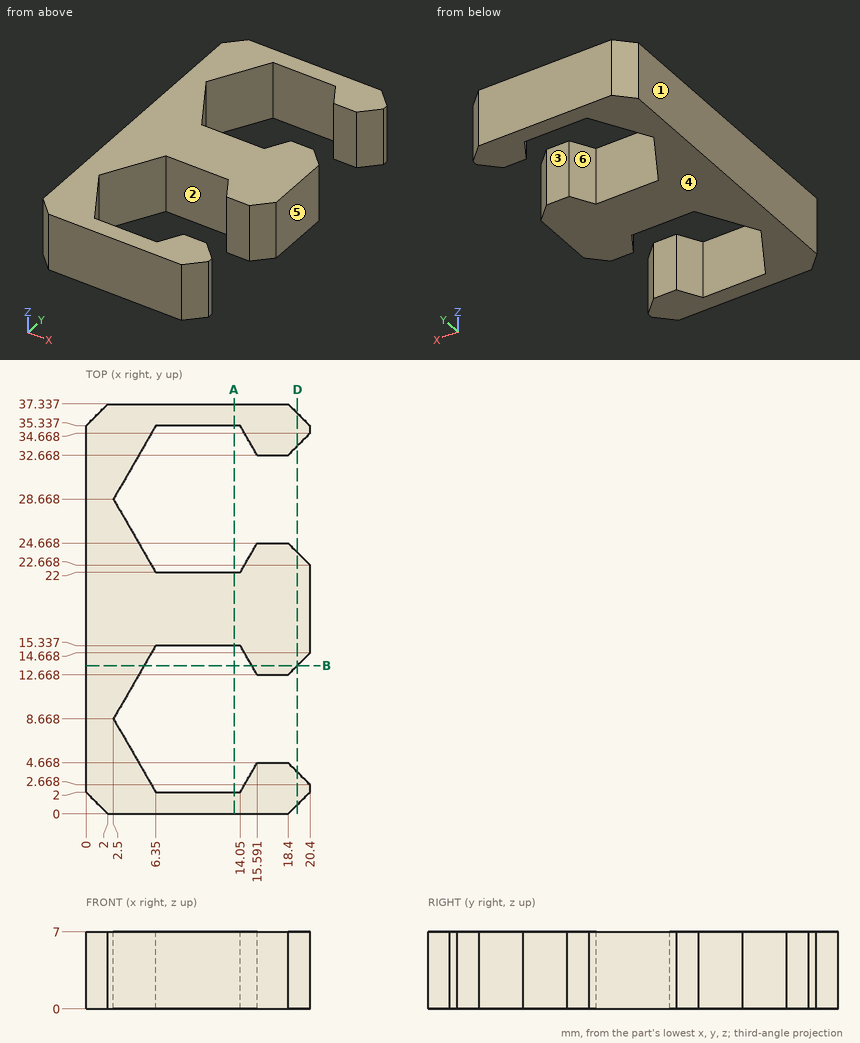
Here's the drawing with two shaded views (mm, measured from the low corner). I have some questions. A direction names the side the tool comes from. Round coordinates to 2 decimals unless told otherwise and drop trailing zeros. Order: outer loops, then holes, each group sorted by start corner. A loop starts at its lowest first (then second) coordinate and runs counter-clockwise, first axis right, second up. Notation, with made-up numbers: (25.25, -23.75) -> (37.25, -23.75) arc R21 cw to (37.25, -2.75) -> close; hole circle Ø7 at (67, 2.5). An arc over 180 degrees is marked (long way). Use a Markdown table: item, result. Add a question column.
(1) For the marked faces 1, 2 and 3, which set-ups out of +Z, -Z, +X, -X, +Y, -Y let a thin tool reach every point of the face, with its end or its side?
(2) Suppose I cut it at A-A, the plane x = 13.5. Please give me the cut outline in (y, z).
(3) For pin 1 Ø1.5 at (y, z) = (10, 5.5) entering from +X; pin 2 Ø6 at (x, y) = (7, 30) entering from +Z; pin 3 Ø1.5 at (y, z) = (5, 3.5) entering from +X, each with a flat end and sliding along its axis, tell me the tip position at first contact or that it passes through.
(4) Suppose I cut it at B-B, the plane y = 13.5. Please give me the cut outline in (x, z).
(5) I need wall thicknesses on line 1 along Y through (x, z) = (10, 2.5); line 2 along Y through (x, z) = (18, 3.5); line 3 along X through (y, z) = (35, 3.5) (1 decimal). Which ranges of each line are inside material? Lowest first, please.
(6) If we mould it in two halves opening along X, with no side actions, what happens to the marked faces 4, 5 and 6? For each: released by +X, released by -X, zero draft, split by the parting line, or undercut.
(7) Suppose I cut it at D-D, the plane x = 19.25. Please give me the cut outline in (y, z), and give its area (3 significant figures).
Verdict:
| question | item | result |
|---|---|---|
| 1 | face 1 | +Z, -Z, -X, +Y, -Y |
| 1 | face 2 | +Z, -Z |
| 1 | face 3 | +Z, -Z, +X |
| 2 | outline | (0, 0) -> (2, 0) -> (2, 7) -> (0, 7) -> close; (15.34, 0) -> (22, 0) -> (22, 7) -> (15.34, 7) -> close; (35.34, 0) -> (37.34, 0) -> (37.34, 7) -> (35.34, 7) -> close |
| 3 | pin 1 | x = 3.7 |
| 3 | pin 2 | through |
| 3 | pin 3 | x = 18.82 |
| 4 | outline | (0, 0) -> (5.29, 0) -> (5.29, 7) -> (0, 7) -> close; (15.11, 0) -> (19.23, 0) -> (19.23, 7) -> (15.11, 7) -> close |
| 5 | line 1 | 0 to 2, 15.34 to 22, 35.34 to 37.34 |
| 5 | line 2 | 0 to 4.67, 12.67 to 24.67, 32.67 to 37.34 |
| 5 | line 3 | 0 to 6.2, 14.2 to 20.4 |
| 6 | face 4 | zero draft |
| 6 | face 5 | released by +X |
| 6 | face 6 | undercut |
| 7 | outline | (0.85, 0) -> (3.82, 0) -> (3.82, 7) -> (0.85, 7) -> close; (13.52, 0) -> (23.82, 0) -> (23.82, 7) -> (13.52, 7) -> close; (33.52, 0) -> (36.49, 0) -> (36.49, 7) -> (33.52, 7) -> close |
| 7 | area | 114 mm2 |
